from build123d import *

# Parameters (mm, degrees)
F1_DEPTH = 50
F2_R     = 7.9375
F3_DEPTH = 98.9010001


# Not quite as in the source:
# - the dataset's text gives a spline's control points without its knots; the knots are read off the source's solid


with BuildPart() as f1:
    # F0 (on Right) → F1 (new body)
    with BuildSketch(Plane.YZ):
        Polygon((0, 5), (0, 0), (317.0611265182, 0), (381, 0), (381, 5), align=None)
        with BuildLine():
            Line((381, 0), (317.0611265182, 0))
            add(Edge.make_bspline(
                [(177.8, -88.9), (248.9784660816, -88.9), (248.9784660816, 0), (317.0611265182, 0)],
                knots=[0, 0, 0, 0, 165.2176484493, 165.2176484493, 165.2176484493, 165.2176484493], degree=3))
            Line((177.8, -88.9), (0, -88.9))
            Line((0, -88.9), (0, -93.9))
            Line((0, -93.9), (177.8, -93.9))
            add(Edge.make_bspline(
                [(177.8, -93.9), (182.5088568902, -93.9), (191.4045001846, -93.163983571), (203.303724493, -90.0815735434), (213.8561143205, -85.3057917839), (223.1918502865, -79.1733759879), (231.500279729, -72.0263439941), (241.5096982859, -61.5630106154), (252.6106670588, -47.4521159829), (263.297288811, -33.7461247303), (272.3524018342, -24.0513036385), (279.564351284, -17.6529202199), (287.3719173686, -12.3368323414), (295.9847641829, -8.2781357767), (305.6793231482, -5.6490337962), (313.0779947533, -5), (317.0611265182, -5)],
                knots=[0, 0, 0, 0, 0.0625, 0.125, 0.1875, 0.25, 0.3125, 0.375, 0.5, 0.625, 0.6875, 0.75, 0.8125, 0.875, 0.9375, 1, 1, 1, 1], degree=3))
            Line((317.0611265182, -5), (381, -5))
            Line((381, -5), (381, 0))
        make_face()
    extrude(amount=-F1_DEPTH)

    # F2 (on face) → F3 (cut, through all)
    with BuildSketch(Plane.XY.offset(5)):
        with Locations((-25, 361.95)):
            Circle(F2_R)
        with Locations((-25, 19.05)):
            Circle(F2_R)
    extrude(amount=-F3_DEPTH, mode=Mode.SUBTRACT)


solid = f1.part
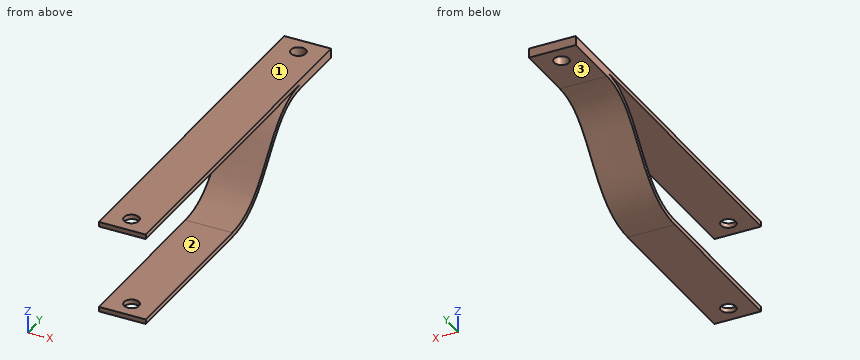
Could you check a few things on this model? Use its own coordinates, in mm. Face numbers are marked on the shaded views. Coordinates: 2 decimals unless noted, no trailing zeros. Write each loop counter-clockwise with the first axis right and the second up, starting at its lowest first coordinate (ties: lowest second). Pieces come first, ordered by that corner, then holes. Notation, with made-up numbers: (2, -7.75) - (56, -7.75) arc R25 cw to (56, 13.25) - close; hole circle Ø6 at (-34.5, 1). An arc over 180 degrees is marked (long way). Put each result on its own line as item: value. Start each with the question number.
Q1. Thinking about a two-plate mould opening in Z: for the marked faces 1, 2 and 3, which applies, pulls with the +Z half, pulls with the -Z half, needs draft (parallel to the pull), parting line crosses it, or undercut?
Q2. I want a section at A-A on y = 19.05. Write out the boundary of the cut face in (x, z), plus the area to 3 significant figures.
Q3. I want a section at C-C on x = -25. Count the separate pieces of the cut face and the enclosed holes in it, plus the area to 3 significant figures.
Q4. I want a section at D-D on y = 361.95. Write out the boundary of the cut face in (x, z).
Q5. I'm going to push flat-ended pins straight in: P1, Ø2, axis at x = -11.5, y = 261.5, coming from the -Z side; P2, Ø8, axis at x = -6.5, z = -47, coming from the -Y side; P3, Ø6, axis at x = -37.5, z = -79, coming from the +Y side. Where does each tip first touch, or does it pass through?
Q6. Please list where these lines run through material, in increasing order: L1, parallel to Z at x = -10, y = 157.5; L2, parallel to Y at x = -25, z = 3; L3, parallel to Z at x = -5.5, y = 181.
Q7. I want a section at B-B on y = 66. Write out the boundary of the cut face in (x, z).
Checks:
1. face 1: pulls with the +Z half
1. face 2: undercut
1. face 3: pulls with the -Z half
2. outline: (-50, -93.9) - (-32.94, -93.9) - (-32.94, -88.9) - (-50, -88.9) - close; (-50, 0) - (-32.94, 0) - (-32.94, 5) - (-50, 5) - close; (-17.06, -93.9) - (0, -93.9) - (0, -88.9) - (-17.06, -88.9) - close; (-17.06, 0) - (0, 0) - (0, 5) - (-17.06, 5) - close
2. area: 341 mm²
3. separate pieces: 4
3. enclosed holes: 0
3. area: 3,660 mm²
4. outline: (-50, -5) - (-32.94, -5) - (-32.94, 5) - (-50, 5) - close; (-17.06, -5) - (0, -5) - (0, 5) - (-17.06, 5) - close
5. P1: z = -37.48
5. P2: y = 243.42
5. P3: y = 226.79
6. L1: -93.9 to -88.9, 0 to 5
6. L2: 0 to 11.11, 26.99 to 354.01, 369.89 to 381
6. L3: -93.84 to -88.84, 0 to 5
7. outline: (-50, -93.9) - (0, -93.9) - (0, -88.9) - (-50, -88.9) - close; (-50, 0) - (0, 0) - (0, 5) - (-50, 5) - close
